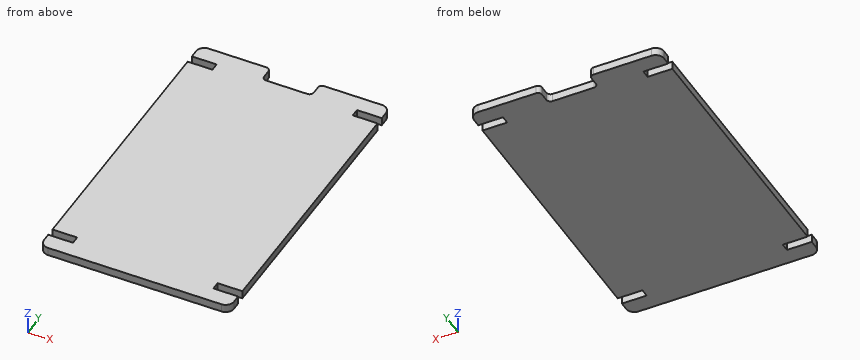
from build123d import *

# Parameters (mm, degrees)
BOSS_EXTRUDE1_DEPTH = 2


with BuildPart() as part:
    # Sketch1 → Boss-Extrude1 (new body)
    with BuildSketch(Plane.XY):
        with BuildLine():
            Line((-21, 38), (-7, 38))
            ThreePointArc((-7, 38), (-6.292893219, 37.707106781), (-6, 37))
            Line((-6, 37), (-6, 35))
            ThreePointArc((-6, 35), (-5.707106781, 34.292893219), (-5, 34))
            Line((-5, 34), (5, 34))
            ThreePointArc((5, 34), (5.707106781, 34.292893219), (6, 35))
            Line((6, 35), (6, 37))
            ThreePointArc((6, 37), (6.292893219, 37.707106781), (7, 38))
            Line((7, 38), (21, 38))
            ThreePointArc((21, 38), (22.414213562, 37.414213562), (23, 36))
            Line((23, 36), (23, 34))
            Line((23, 34), (17, 34))
            Line((17, 34), (17, 32))
            Line((17, 32), (23, 32))
            Line((23, 32), (23, -32))
            Line((23, -32), (17, -32))
            Line((17, -32), (17, -34))
            Line((17, -34), (23, -34))
            Line((23, -34), (23, -36))
            ThreePointArc((23, -36), (22.414213562, -37.414213562), (21, -38))
            Line((21, -38), (-21, -38))
            ThreePointArc((-21, -38), (-22.414213562, -37.414213562), (-23, -36))
            Line((-23, -36), (-23, -34))
            Line((-23, -34), (-17, -34))
            Line((-17, -34), (-17, -32))
            Line((-17, -32), (-23, -32))
            Line((-23, -32), (-23, 32))
            Line((-23, 32), (-17, 32))
            Line((-17, 32), (-17, 34))
            Line((-17, 34), (-23, 34))
            Line((-23, 34), (-23, 36))
            ThreePointArc((-23, 36), (-22.414213562, 37.414213562), (-21, 38))
        make_face()
    extrude(amount=BOSS_EXTRUDE1_DEPTH)


solid = part.part
Could you check a few things on this model? Use its own coordinates, in mm. Round coordinates to 2 decimals unless told otherwise and drop trailing zeros. Write each loop counter-clockwise with the first axis right and the second up, starting at its lowest first coordinate (ties: lowest second). Pieces come first, ordered by that corner, then holes. Notation, with made-up numbers: (66.5, 52.5) - (114.5, 52.5) arc R26 ccw to (114.5, 66.5) - close; hole circle Ø6 at (48, 26). An arc over 180 degrees is marked (long way). Put each result on its own line as item: value. Start each with the question number.
(1) I want a section at C-C, the plane x = 0. Please give me the cut outline in (y, z).
(2) I want a section at A-A, the plane x = -19. Please give me the cut outline in (y, z), plus the area to 3 significant figures.
(3) Will these pins go through, and if not, where does the flat tip stop? pin 1 (0.6 mm diameter, centred on y = -32.5, z = 1, fed in from -X); pin 2 (0.6 mm diameter, centred on y = 33, z = 0.5, fed in from +X); pin 3 (1 mm diameter, centred on x = 21.5, z = 1, fed in from -Y).
(4) I need wall thicknesses on probe 1 along Y at (x, z) = (-18.5, 0.5); probe 2 along Y at (x, z) = (2, 0.65). Which ranges of each line are inside material? Lowest first, please.
Here are the results:
1. outline: (-38, 0) - (34, 0) - (34, 2) - (-38, 2) - close
2. outline: (-38, 0) - (-34, 0) - (-34, 2) - (-38, 2) - close; (-32, 0) - (32, 0) - (32, 2) - (-32, 2) - close; (34, 0) - (38, 0) - (38, 2) - (34, 2) - close
2. area: 144 mm^2
3. pin 1: stops at x = -17
3. pin 2: stops at x = 17
3. pin 3: stops at y = -38
4. probe 1: y = -38 to -34, -32 to 32, 34 to 38
4. probe 2: y = -38 to 34
